from build123d import *

# Parameters (mm, degrees)
F0_R      = 13
F5_DEPTH  = 20
F4_R      = 8.6
F6_DEPTH  = 23
F3_R      = 3.3
F8_DEPTH  = 8
F9_DEPTH  = 12
F10_R     = 2.05
F11_DEPTH = 15
F12_R     = 1.5
F13_DEPTH = 25
F15_R     = 3.5
F16_DEPTH = 5
F19_DEPTH = 3


with BuildPart() as f5:
    # F0 (on Top) → F5 (new body, symmetric)
    with BuildSketch(Plane.XY):
        Circle(F0_R)
    extrude(amount=F5_DEPTH, both=True)

    # F4 (on offset) → F6 (cut)
    with BuildSketch(Plane.XY.offset(-20)):
        Circle(F4_R)
    extrude(amount=F6_DEPTH, mode=Mode.SUBTRACT)

    # F3 (on offset) → F8 (cut)
    with BuildSketch(Plane.XY.offset(20)):
        with Locations((0.0063437128, 0)):
            Circle(F3_R)
    extrude(amount=-F8_DEPTH, mode=Mode.SUBTRACT)

    # F7 (on Top) → F9 (cut)
    with BuildSketch(Plane.XY):
        with BuildLine():
            Line((1.888, 2.9471097706), (0, 2.9471097706))
            Line((0, 2.9471097706), (-1.888, 2.9471097706))
            ThreePointArc((-1.888, 2.9471097706), (0, -3.5), (1.888, 2.9471097706))
        make_face()
    extrude(amount=F9_DEPTH, mode=Mode.SUBTRACT)

    # F10 (on Right) → F11 (cut, symmetric)
    with BuildSketch(Plane.YZ):
        with Locations((-2.5, -12.5)):
            Circle(F10_R)
    extrude(amount=F11_DEPTH, both=True, mode=Mode.SUBTRACT)

    # F12 (on Front) → F13 (cut)
    with BuildSketch(Plane.XZ):
        with Locations((0, 7)):
            Circle(F12_R)
    extrude(amount=-F13_DEPTH, mode=Mode.SUBTRACT)

    # F15 (on offset) → F16 (cut)
    with BuildSketch(Plane.YZ.offset(11)):
        with Locations((-2.5, -12.5)):
            Circle(F15_R)
    extrude(amount=F16_DEPTH, mode=Mode.SUBTRACT)

    # F18 (on offset) → F19 (cut)
    with BuildSketch(Plane.YZ.offset(-12)):
        Polygon((-5.9460342998, -10.8984858401), (-5.6099690969, -14.683596166), (-2.1639347971, -16.2851103259), (0.9460342998, -14.1015141599), (0.6099690969, -10.316403834), (-2.8360652029, -8.7148896741), align=None)
    extrude(amount=-F19_DEPTH, mode=Mode.SUBTRACT)


solid = f5.part
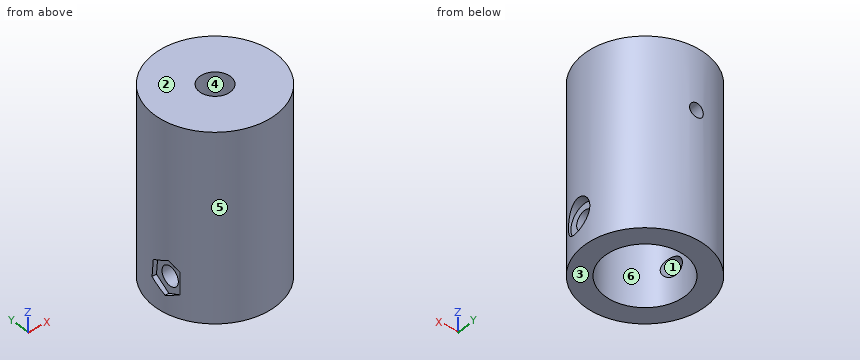
Part model, mm, in its own coordinate system. Face numbers are marked on the shaded views. A direction names the side the tool comes from. Coordinates: 2 decimals unless noted, no trailing zeros. Loops run counter-clockwise (first coordinate to the right, second up) from the corner with the lowest first, then second, coordinate; pieces in that order, holes last. Notation, with made-up numbers: (68, 42.5) - (123, 42.5) arc R17 cw to (123, 57.5) - close; hole circle Ø5 at (22, 21.25). An arc over 180 degrees is marked (long way). Write each question's results on one line, items separated by ' | '. Start each with the question number.
Q1. Probe line 1 along X through (y, z) = (0, 8); line 2 along Y through (x, z) = (0, -9); line 3 along Z through (x, y) = (-9, -2.5). List the from-to ranges inside material, lowest first.
Q2. Two-plate mould, pull along Z, no slides. Class the marked faces 1, 2, 3 and 4: +Z half, -Z half, draft (parallel to the pull), parting line (faces both ways), or undercut.
Q3. Slice it at B-B on y = 0. Give the cut face in (x, z), and give its area (3 significant figures).
Q4. Slice it at C-C on z = 1.5. Give the cut face in (x, y), and give its area (3 significant figures).
Q5. Which spindle directions (+Z, -Z, +X, -X, +Y, -Y) get a long thin tool onto all of the face, cutting with end or side? Do the marked faces 5 and 6. Say none if no direction does.
Q6. Drop flat-ended pins along their axis: pin 1 Ø5 at (x, y) = (-1.5, 0) entering from -Z; pin 2 Ø4.5 at (y, z) = (-2.5, -12.5) entering from -X; pin 3 Ø5.5 at (y, z) = (-2.5, -12) entering from +X; pin 4 Ø5.5 at (x, y) = (0, 0) entering from -Z. Give the stop position or say it passes through.
Q7. Slice it at D-D on y = 11.25. Give the cut face in (x, z), and give its area (3 significant figures).
Q8. Slice it at A-A on z = -13.5. Give the cut face in (x, y), and give its area (3 significant figures).
Answer:
1) line 1: x = -13 to -3.5, 3.5 to 13 | line 2: y = -13 to -8.6, 8.6 to 13 | line 3: z = -20 to -14.55, -10.45 to 20
2) face 1: undercut | face 2: +Z half | face 3: -Z half | face 4: draft
3) outline: (-13, -20) - (-8.6, -20) - (-8.6, 3) - (-3.5, 3) - (-3.5, 12) - (-3.29, 12) - (-3.29, 20) - (-13, 20) - (-13, -10.03) - (-12, -10.03) - (-12, -14.77) - (-13, -14.77) - close; (3.31, 12) - (3.5, 12) - (3.5, 3) - (8.6, 3) - (8.6, -20) - (13, -20) - (13, -14.95) - (11, -14.95) - (11, -10.05) - (13, -10.05) - (13, 20) - (3.31, 20) - close | area: 514 mm2
4) outline: circle Ø26 at (0, 0); hole circle Ø17.2 at (0, 0) | area: 299 mm2
5) face 5: +Z, -Z | face 6: -Z
6) pin 1: stops at z = 3 | pin 2: stops at x = -12 | pin 3: stops at x = 11 | pin 4: passes through
7) outline: (-6.51, -20) - (6.51, -20) - (6.51, 20) - (-6.51, 20) - close; hole circle Ø3 at (0, 7) | area: 514 mm2
8) outline: (-12.97, 0.89) - (-12, 0.89) - (-12, -0.71) - (-8.57, -0.71) arc R8.6 cw (long way) to (8.57, -0.71) - (11, -0.71) - (11, 0.85) - (12.97, 0.85) arc R13 ccw to start; (-12, -5) arc R13 ccw to (11.61, -5.85) - (11, -5.85) - (11, -4.29) - (7.45, -4.29) arc R8.6 cw to (-7.45, -4.29) - (-12, -4.29) - close | area: 260 mm2
